Can you work these out from the model? Positions are in its coordinate system, mm. Round coordinates to 2 decimals unless told otherwise and drop trailing zeros. Loops run counter-clockwise (first coordinate to the right, second up) from the corner with the lowest first, then second, coordinate; pieces in that order, holes last. Notation, with made-up numbers: (7, 6.25) -> (30, 6.25) arc R24 ccw to (30, 24.25) -> close; hole circle Ø10 at (25, 19). An arc over 180 degrees is marked (long way). Write item = value, one per line.
Autodesk Inventor part; units mm, degrees
ref_plane "YZ Plane" through (0, 0, 0) normal (1, 0, 0) x (0, 1, 0)
ref_plane "XZ Plane" through (0, 0, 0) normal (0, 1, 0) x (-1, 0, 0)
ref_plane "XY Plane" through (0, 0, 0) normal (0, 0, 1) x (1, 0, 0)
sketch "Sketch1" plane through (0, 0, 0) normal (0, 0, 1) x (1, 0, 0)
  line L0 (0, 0) -> (3.7042, 0)
  line L1 (1.8521, 0) -> (1.8521, 0.6615)
  line L2 (1.8521, 0.6615) -> (2.1167, 0.6615)
  line L3 (2.1167, 0.6615) -> (3.7042, 0.295)
  line L4 (3.7042, 0.295) -> (3.7042, 0)
  line L5 (1.8521, 0.6615) -> (1.8521, 2.7781)
  line L6 (1.8521, 2.7781) -> (2.1167, 2.7781)
  line L7 (2.1167, 2.7781) -> (2.1167, 0.6615)
  line L8 (1.8521, 2.7781) -> (1.8521, 3.8365)
  line L9 (1.8521, 3.8365) -> (2.8549, 3.8365)
  line L10 (2.1167, 2.7781) -> (3.1089, 3.0072)
  line L11 (2.1167, 2.7781) -> (3.135, 2.7781) construction
  line L12 (3.1089, 3.5825) -> (3.1089, 3.0072)
  arc A0 (3.1089, 3.5825) -> (2.8549, 3.8365) centre (2.8549, 3.5825) ccw
  line L13 (3.7042, 0) -> (0, 0)
  line L14 (1.8521, 0.6615) -> (1.5875, 0.6615)
  line L15 (1.5875, 0.6615) -> (0, 0.295)
  line L16 (0, 0.295) -> (0, 0)
  line L17 (1.8521, 2.7781) -> (1.5875, 2.7781)
  line L18 (1.5875, 2.7781) -> (1.5875, 0.6615)
  line L19 (1.8521, 3.8365) -> (0.8493, 3.8365)
  line L20 (1.5875, 2.7781) -> (0.5953, 3.0072)
  line L21 (1.5875, 2.7781) -> (0.5692, 2.7781) construction
  line L22 (0.5953, 3.5825) -> (0.5953, 3.0072)
  arc A1 (0.8493, 3.8365) -> (0.5953, 3.5825) centre (0.8493, 3.5825) ccw
  dimension "d3" = 0.6615
  dimension "d4" = 0.2646
  dimension "d5" = 167
  dimension "d6" = 2.1167
  dimension "d7" = 1.0583
  dimension "d9" = 13
  dimension "d10" = 0.254
extrude "Extrusion1" add sketch "Sketch1" against normal blind 127
properties part number "Rail48in"
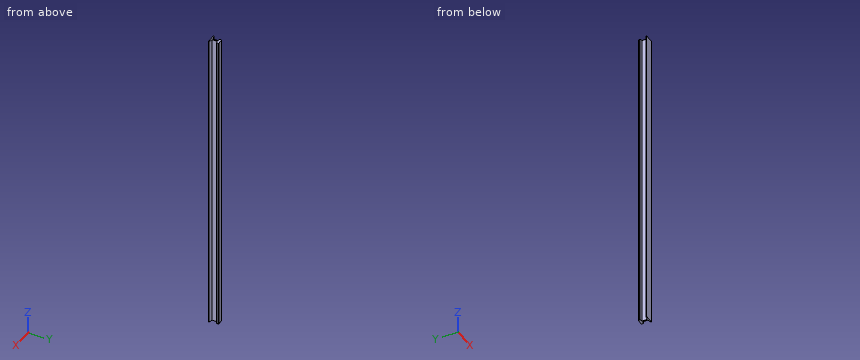
1. I'm going to push flat-ended pins straight in: pin 1 (0.6 mm diameter, centred on y = 3.5, z = -40.5, fed in from -X); pin 2 (1.1 mm diameter, centred on y = 1.5, z = -46, fed in from +X); pin 3 (0.5 mm diameter, centred on y = 3.5, z = -56, fed in from +X). Where does each tip first touch, or does it pass through?
Entries:
pin_1 = 0.6
pin_2 = 2.12
pin_3 = 3.11
2. Suppose I cut it at B-B, the plane y = 1.85. List the corners of the cut face in (x, z) for me.
Entries:
outline = (1.59, -127) -> (2.12, -127) -> (2.12, 0) -> (1.59, 0) -> close
3. I need wall thicknesses on line 1 (X direction, y = 1.35, z = -98); line 2 (Y direction, x = 2.2, z = -53.5); line 3 (Y direction, x = 1, z = -89.5). Which ranges of each line are inside material? Lowest first, please. Write a range as [from, to].
Entries:
line_1 = [1.59, 2.12]
line_2 = [0, 0.64], [2.8, 3.84]
line_3 = [0, 0.53], [2.91, 3.84]
